```python
from build123d import *

# Parameters (mm, degrees)
BOSS_EXTRUDE1_DEPTH      = 33.2
BOSS_EXTRUDE2_DEPTH      = 5
BOSS_EXTRUDE2_DEPTH_BACK = 5
SKETCH4_W                = 83.511672616
SKETCH4_H                = 9.134615549
SKETCH5_R                = 32
BOSS_EXTRUDE3_DEPTH      = 5
SKETCH6_R                = 2.5
CUT_EXTRUDE1_DEPTH       = 5


with BuildPart() as part:
    # Sketch2 → Boss-Extrude1 (new body)
    with BuildSketch(Plane(origin=(0, 0, 0), x_dir=(1, 0, 0), z_dir=(0, 1, 0))):
        with BuildLine():
            ThreePointArc((-143.85, -86.4), (-135.063203436, -107.613203436), (-113.85, -116.4))
            Line((-113.85, -116.4), (113.85, -116.4))
            ThreePointArc((113.85, -116.4), (135.063203436, -107.613203436), (143.85, -86.4))
            Line((143.85, -86.4), (143.85, 86.4))
            ThreePointArc((143.85, 86.4), (135.063203436, 107.613203436), (113.85, 116.4))
            Line((113.85, 116.4), (-113.85, 116.4))
            ThreePointArc((-113.85, 116.4), (-135.063203436, 107.613203436), (-143.85, 86.4))
            Line((-143.85, 86.4), (-143.85, -86.4))
        make_face()
    extrude(amount=BOSS_EXTRUDE1_DEPTH)



with BuildPart() as body_2:
    # Sketch3 → Revolve2 (revolve)
    with BuildSketch(Plane(origin=(39.95, 0, 0), x_dir=(0, 0, -1), z_dir=(1, 0, 0))):
        Polygon((85.6, -30.3), (85.6, -5.3), (-1.35, -5.3), (-88.3, -17.8), (-88.3, -30.3), align=None)
    revolve(axis=Axis((39.95, -30.3, -85.6), (0, 0, 1)))


with BuildPart() as part_1:
    add(part.part)

    add(body_2.part)  # Boss-Extrude2 merges body 2
    # Sketch4 → Boss-Extrude2 (add, two sides: drawn at the far end of the back side and taken through both)
    with BuildSketch(Plane(origin=(39.95, 0, 0), x_dir=(0, 0, -1), z_dir=(1, 0, 0)).offset(-BOSS_EXTRUDE2_DEPTH_BACK)):
        with Locations((41.755836308, -4.567307775)):
            Rectangle(SKETCH4_W, SKETCH4_H)
    extrude(amount=BOSS_EXTRUDE2_DEPTH + BOSS_EXTRUDE2_DEPTH_BACK)

    # Sketch5 → Boss-Extrude3 (add)
    with BuildSketch(Plane.XZ):
        with Locations(Location((-108.35, -70, 0), (0, 0, 90))):
            Circle(SKETCH5_R)
    extrude(amount=BOSS_EXTRUDE3_DEPTH)

    # Sketch6 → Cut-Extrude1 (cut)
    with BuildSketch(Plane.XZ):
        with Locations(Location((113.85, -86.4, 0), (0, 0, 270))):
            Circle(SKETCH6_R)
        with Locations(Location((0, -86.4, 0), (0, 0, 270))):
            Circle(SKETCH6_R)
        with Locations(Location((113.85, 86.4, 0), (0, 0, 270))):
            Circle(SKETCH6_R)
        with Locations(Location((0, 86.4, 0), (0, 0, 270))):
            Circle(SKETCH6_R)
        with Locations(Location((-113.85, 86.4, 0), (0, 0, 270))):
            Circle(SKETCH6_R)
    extrude(amount=-CUT_EXTRUDE1_DEPTH, mode=Mode.SUBTRACT)


solid = part_1.part
```
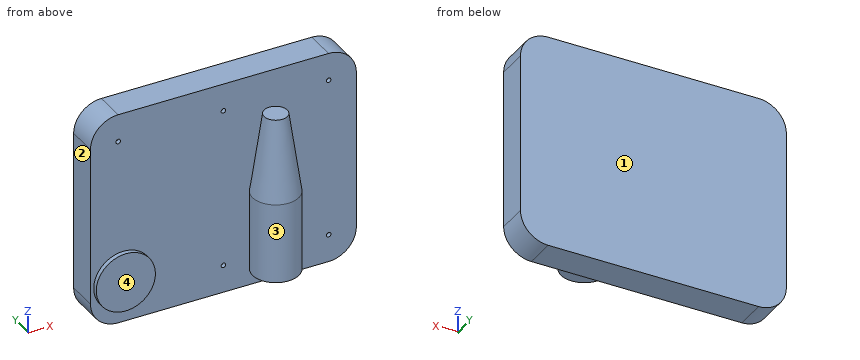
Can you work these out from the model? Positions are in its coordinate system, mm. Face numbers are marked on the shaded views. Give positions to 0.01 mm unless a question says otherwise; leave off trailing zeros. Order: outer loops, then holes, each group sorted by start corner. A loop starts at its lowest first (then second) coordinate and runs counter-clockwise, first axis right, second up. Notation, with made-up numbers: (62.25, 25.25) - (94.25, 25.25) arc R30 cw to (94.25, 62.25) - close; hole circle Ø1 at (59, 31.5). An arc over 180 degrees is marked (long way). Use a Markdown table: item, result. Add a question column.
Q1. If we section it at A-A on z = -21: Write out the boundary of the cut face in (x, y), plus the area to 3 significant figures.
Q2. If we section it at C-C on z = 44.5: Write out the boundary of the cut face in (x, y).
Q3. If we mould it in two halves opening along Y, with no side actions, what happens to the marked faces 1, 2, 3 and 4? For each: released by +Y, released by -Y, zero draft, split by the parting line, or undercut.
Q4. Please list where these lines run through material, in increasing order: line 1 along X through (y, z) = (1.9, -86.4); line 2 along X through (y, z) = (2.2, 86.4); line 3 along Y through (x, z) = (73, -91.5).
Q5. I'm going to push flat-ended pins straight in: pin 1 (5.5 mm diameter, centred on x = 113.5, z = 86, fed in from -Y); pin 2 (15 mm diameter, centred on x = 48.5, y = -43, fed in from -Z); pin 3 (1.5 mm diameter, centred on x = 0.5, z = -87.5, fed in from -Y). Where does each tip first touch, or does it pass through?
Q6. If we section it at D-D on z = -70: Write out the boundary of the cut face in (x, y).
Q7. If we section it at B-B on x = 39.95: Write out the boundary of the cut face in (y, z), plus the area to 3 significant figures.
Answers follow:
| question | item | result |
|---|---|---|
| 1 | outline | (-143.85, 0) - (34.95, 0) - (34.95, -5.81) arc R25 ccw (long way) to (44.95, -5.81) - (44.95, 0) - (143.85, 0) - (143.85, 33.2) - (-143.85, 33.2) - close |
| 1 | area | 11,600 mm^2 |
| 2 | outline | (-143.85, 0) - (143.85, 0) - (143.85, 33.2) - (-143.85, 33.2) - close; circle Ø37.59 at (39.95, -30.3) |
| 3 | face 1 | released by +Y |
| 3 | face 2 | zero draft |
| 3 | face 3 | undercut |
| 3 | face 4 | released by -Y |
| 4 | line 1 | x = -143.85 to -2.5, 2.5 to 111.35, 116.35 to 143.85 |
| 4 | line 2 | x = -143.85 to -116.35, -111.35 to -2.5, 2.5 to 111.35, 116.35 to 143.85 |
| 4 | line 3 | y = 0 to 33.2 |
| 5 | pin 1 | stops at y = 0 |
| 5 | pin 2 | stops at z = -85.6 |
| 5 | pin 3 | stops at y = 5 |
| 6 | outline | (-143.85, 0) - (-140.35, 0) - (-140.35, -5) - (-76.35, -5) - (-76.35, 0) - (34.95, 0) - (34.95, -5.81) arc R25 ccw (long way) to (44.95, -5.81) - (44.95, 0) - (143.85, 0) - (143.85, 33.2) - (-143.85, 33.2) - close |
| 7 | outline | (-55.3, -85.6) - (-5.3, -85.6) - (-5.3, -83.51) - (0, -83.51) - (0, -116.4) - (33.2, -116.4) - (33.2, 116.4) - (0, 116.4) - (0, 0) - (-5.3, 0) - (-5.3, 1.35) - (-17.8, 88.3) - (-42.8, 88.3) - (-55.3, 1.35) - close |
| 7 | area | 15,800 mm^2 |
